Autodesk Inventor part; units mm, degrees
ref_plane "YZ Plane" through (0, 0, 0) normal (1, 0, 0) x (0, 1, 0)
ref_plane "XZ Plane" through (0, 0, 0) normal (0, 1, 0) x (-1, 0, 0)
ref_plane "XY Plane" through (0, 0, 0) normal (0, 0, 1) x (1, 0, 0)
sketch "Sketch1" plane through (0, 0, 0) normal (0, 0, 1) x (1, 0, 0)
  circle A0 centre (0, 0) radius 6
  line L0 (-13, 13) -> (13, 13)
  line L1 (13, 13) -> (13, -13)
  line L2 (13, -13) -> (-13, -13)
  line L3 (-13, -13) -> (-13, 13)
  line L4 (0, 0) -> (13, 13)
  line L5 (6.5, 6.5) -> (13, 13)
  circle A1 centre (9.75, 9.75) radius 0.5
  line L6 (0, 0) -> (-13, 13)
  line L7 (-6.5, 6.5) -> (-13, 13)
  circle A2 centre (-9.75, 9.75) radius 0.5
  line L8 (0, 0) -> (-13, -13)
  line L9 (-6.5, -6.5) -> (-13, -13)
  circle A3 centre (-9.75, -9.75) radius 0.5
  line L10 (0, 0) -> (13, -13)
  line L11 (6.5, -6.5) -> (13, -13)
  circle A4 centre (9.75, -9.75) radius 0.5
  line L12 (-5, -13) -> (5, -13)
  line L13 (5, -13) -> (5, -9.5)
  line L14 (5, -9.5) -> (-5, -9.5)
  line L15 (-5, -9.5) -> (-5, -13)
  line L16 (13, 5) -> (9.5, 5)
  line L17 (9.5, 5) -> (9.5, -5)
  line L18 (9.5, -5) -> (13, -5)
  line L19 (-5, 13) -> (-5, 9.5)
  line L20 (-5, 9.5) -> (5, 9.5)
  line L21 (5, 9.5) -> (5, 13)
  line L22 (-13, -5) -> (-9.5, -5)
  line L23 (-9.5, -5) -> (-9.5, 5)
  line L24 (-9.5, 5) -> (-13, 5)
  point P0 (0, 13)
  point P1 (13, 0)
  point P2 (0, -9.5)
  point P3 (0, -13)
  point P4 (9.5, 0)
  point P5 (0, 9.5)
  point P6 (-9.5, 0)
  dimension "d0" = 12
  dimension "d1" = 26
  dimension "d2" = 26
  dimension "d3" = 1
  dimension "d6" = 360
  dimension "d10" = 10
  dimension "d11" = 3.5
  dimension "d14" = 360
extrude "Extrusion1" add sketch "Sketch1" along normal mid plane 3.5 contours A0 L4 A1 L1 L16 L17 L18 L10 A4 | A0 L6 A2 L0 L19 L20 L21 L4 A1 | L10 A4 L2 L13 L14 L15 L8 A3 A0 | A0 L8 A3 L3 L22 L23 L24 L6 A2
equation "\"d2\" = d1"
properties part number "Spodnji del - Drzalo za pismo"
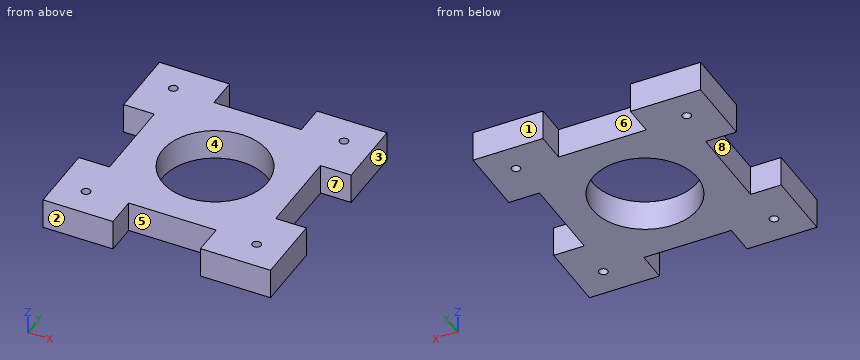
The model under review builds one solid part; all positions refer to its coordinate system, in mm. Face numbers are marked on the shaded views. A direction names the side the tool comes from. Round coordinates to 2 decimals unless told otherwise and drop trailing zeros. Write each loop counter-clockwise with the first axis right and the second up, starting at its lowest first coordinate (ties: lowest second). Pieces come first, ordered by that corner, then holes. Notation, with made-up numbers: (12.25, 66) -> (63.25, 66) arc R23 ccw to (63.25, 91) -> close; hole circle Ø1 at (21.5, 55.5). An arc over 180 degrees is marked (long way). Answer as a JSON object with one key per item and string values.
1. We need section A-A on y = -11. State the section outline as (x, z) points, and give its area (3 significant figures).
Results found:
{"outline": "(-13, -1.75) -> (-5, -1.75) -> (-5, 1.75) -> (-13, 1.75) -> close; (5, -1.75) -> (13, -1.75) -> (13, 1.75) -> (5, 1.75) -> close", "area": "56.0 mm^2"}
2. Machinability: for the marked faces 5, 6, 7 and 8, which of the approach directions +Z, -Z, +X, -X, +Y, -Y give a long, thin tool a straight path to every point of the face, cutting with its end or side? Answer none if there is none.
Results found:
{"face 5": "+Z, -Z, -Y", "face 6": "+Z, -Z, +Y", "face 7": "+Z, -Z, +X", "face 8": "+Z, -Z, -X"}
3. To check wall thickness, follow line 1 along X through (y, z) = (-9.75, -0.5); line 2 along Y through (x, z) = (10.5, -1.5). State the ranges of each line that lie inside material, in increasing order.
Results found:
{"line 1": "x = -13 to -10.25, -9.25 to -5, 5 to 9.25, 10.25 to 13", "line 2": "y = -13 to -5, 5 to 13"}
4. We need section C-C on z = -1.35. State the section outline as (x, y) points, and give its area (3 significant figures).
Results found:
{"outline": "(-13, -13) -> (-5, -13) -> (-5, -9.5) -> (5, -9.5) -> (5, -13) -> (13, -13) -> (13, -5) -> (9.5, -5) -> (9.5, 5) -> (13, 5) -> (13, 13) -> (5, 13) -> (5, 9.5) -> (-5, 9.5) -> (-5, 13) -> (-13, 13) -> (-13, 5) -> (-9.5, 5) -> (-9.5, -5) -> (-13, -5) -> close; hole circle Ø1 at (-9.75, -9.75); hole circle Ø1 at (-9.75, 9.75); hole circle Ø12 at (0, 0); hole circle Ø1 at (9.75, -9.75); hole circle Ø1 at (9.75, 9.75)", "area": "420 mm^2"}
5. Clearance check with flat-ended pins moving along their axes: pin 1 (1.5 mm diameter, centred on x = -1.5, z = 0, fed in from +Y); pin 2 (1.8 mm diameter, centred on y = 2, z = 0.5, fed in from +X); pin 3 (1.8 mm diameter, centred on x = -1, z = -0.5, fed in from -Y). State where each tip first meets the part, or that it passes through.
Results found:
{"pin 1": "stops at y = 9.5", "pin 2": "stops at x = 9.5", "pin 3": "stops at y = -9.5"}
6. The part is to be moulded in two halves that separate along Y. For the marked faces 1, 2, 3 and 4, say which applies: pulls with the +Y half, pulls with the -Y half, needs draft (parallel to the pull), parting line crosses it, or undercut.
Results found:
{"face 1": "pulls with the +Y half", "face 2": "pulls with the -Y half", "face 3": "needs draft", "face 4": "undercut"}
7. We need section B-B on x = 0. State the section outline as (y, z) points, and give its area (3 significant figures).
Results found:
{"outline": "(-9.5, -1.75) -> (-6, -1.75) -> (-6, 1.75) -> (-9.5, 1.75) -> close; (6, -1.75) -> (9.5, -1.75) -> (9.5, 1.75) -> (6, 1.75) -> close", "area": "24.5 mm^2"}
